```python
from build123d import *

# Parameters (mm, degrees)
SKETCH1_W                = 185
SKETCH1_H                = 70
SKETCH1_W_2              = 225
SKETCH1_H_2              = 30
BOSS_EXTRUDE1_DEPTH      = 380
CUT_EXTRUDE1_START       = -130
CUT_EXTRUDE1_OUTLINE_W   = 225
CUT_EXTRUDE1_OUTLINE_H   = 320
CUT_EXTRUDE1_OUTLINE_W_2 = 185
CUT_EXTRUDE1_DEPTH       = 130
SKETCH3_W                = 320
SKETCH3_H                = 30
CUT_EXTRUDE2_DEPTH       = 30
SKETCH4_W                = 320
SKETCH4_H                = 70
CUT_EXTRUDE3_DEPTH       = 245


# Read off the part's stored shape, not the designer's step: Cut-Extrude1
with BuildPart() as part:
    # Sketch1 → Boss-Extrude1 (new body)
    with BuildSketch(Plane.XY):
        Polygon((250, 25), (-5, 25), (-5, 65), (-250, 65), (-250, -65), (250, -65), align=None)
        with Locations((-127.5, 0)):
            Rectangle(SKETCH1_W, SKETCH1_H, mode=Mode.SUBTRACT)
        with Locations((107.5, -20)):
            Rectangle(SKETCH1_W_2, SKETCH1_H_2, mode=Mode.SUBTRACT)
    extrude(amount=BOSS_EXTRUDE1_DEPTH)

    # Cut-Extrude1 outline → Cut-Extrude1 (cut)
    with BuildSketch(Plane(origin=(0, 65, 0), x_dir=(1, 0, 0), z_dir=(0, 1, 0)).offset(CUT_EXTRUDE1_START)):
        with Locations((107.5, -190)):
            Rectangle(CUT_EXTRUDE1_OUTLINE_W, CUT_EXTRUDE1_OUTLINE_H)
        with Locations((-127.5, -190)):
            Rectangle(CUT_EXTRUDE1_OUTLINE_W_2, CUT_EXTRUDE1_OUTLINE_H)
    extrude(amount=CUT_EXTRUDE1_DEPTH, mode=Mode.SUBTRACT)

    # Sketch3 → Cut-Extrude2 (cut)
    with BuildSketch(Plane(origin=(250, 0, 0), x_dir=(0, 0, -1), z_dir=(1, 0, 0))):
        with Locations((-190, -20)):
            Rectangle(SKETCH3_W, SKETCH3_H)
    extrude(amount=-CUT_EXTRUDE2_DEPTH, mode=Mode.SUBTRACT)

    # Sketch4 → Cut-Extrude3 (cut)
    with BuildSketch(Plane.ZY.offset(250)):
        with Locations((190, 0)):
            Rectangle(SKETCH4_W, SKETCH4_H)
    extrude(amount=-CUT_EXTRUDE3_DEPTH, mode=Mode.SUBTRACT)


solid = part.part
```
Check sheet for the modelled part. Datum: model origin and axes. Units: mm. A direction names the side the tool comes from. Give positions to 0.01 mm unless a question says otherwise; leave off trailing zeros. Loops run counter-clockwise (first coordinate to the right, second up) from the corner with the lowest first, then second, coordinate; pieces in that order, holes last. Notation, with made-up numbers: (-21.75, -33) - (36.25, -33) arc R5 ccw to (36.25, -28) - close; hole circle Ø7 at (32, -3.75). An arc over 180 degrees is marked (long way). One line per question, with ' | ' between items. Start each with the question number.
1. Cross-section at B-B, the plane x = -116.5. Enter the section's corners in (y, z), plus the area to 3 significant figures.
2. Gauge pin test, flat ends, axial feed: pin 1 Ø24 at (x, z) = (87.5, 9) entering from +Y; pin 2 Ø12 at (x, y) = (23, -9.5) entering from +Z; pin 3 Ø4 at (y, z) = (7, 245) entering from -X. Record the tip position at first contact, or that the pin passes through.
3. Cross-section at A-A, the plane z = 313.5. Enter the section's corners in (x, y).
4. Set-up check for faces 1 (the flat face through (-20, -35, 188)), 2 (the flat face through (-129, -50, 30)), 3 (the flat face through (106, -5, 365)), 4 (the flat face through (-250, 44, 187)): record each of +Z, -Z, +X, -X, +Y, -Y from which the full face is reachable in a straight line by a thin tool's end or side.
5. Cross-section at C-C, the plane y = -29. Enter the section's corners in (x, z), plus the area to 3 significant figures.
6. Cross-section at D-D, the plane y = -56. Enter the section's corners in (x, z), plus the area to 3 significant figures.
7. Draft check along Y on faces 5 (the flat face through (-235, -35, 188)), 6 (the flat face through (220, -50, 192)), 7 (the flat face through (-35, 0, 15)), 8 (the flat face through (227, 25, 189)). Enter one of: released by +Y, released by -Y, zero draft, split by the parting line, or undercut.
8. Material ranges on line 1 along X through (y, z) = (-52.5, 209); line 2 along Z through (x, y) = (60, -45); line 3 along Y through (x, z) = (-14, 54), recorded low to high. Write a range as [from, to].
Check result:
1) outline: (-65, 0) - (-35, 0) - (-35, 30) - (-65, 30) - close; (-65, 350) - (-35, 350) - (-35, 380) - (-65, 380) - close; (35, 0) - (65, 0) - (65, 30) - (35, 30) - close; (35, 350) - (65, 350) - (65, 380) - (35, 380) - close | area: 3,600 mm2
2) pin 1: stops at y = 25 | pin 2: stops at z = 380 | pin 3: stops at x = 220
3) outline: (-250, -65) - (-220, -65) - (-220, -35) - (-250, -35) - close; (-250, 35) - (-220, 35) - (-220, 65) - (-250, 65) - close; (-35, -65) - (-5, -65) - (-5, -35) - (-35, -35) - close; (-35, 35) - (-5, 35) - (-5, 65) - (-35, 65) - close; (220, -65) - (250, -65) - (250, -35) - (220, -35) - close; (220, -5) - (250, -5) - (250, 25) - (220, 25) - close
4) face 1: +X, -X | face 2: +Y, -Y | face 3: +Z, -Z | face 4: +Z, -Z, -X, +Y, -Y
5) outline: (-250, 0) - (-220, 0) - (-220, 30) - (-250, 30) - close; (-250, 350) - (-220, 350) - (-220, 380) - (-250, 380) - close; (-35, 0) - (-5, 0) - (-5, 30) - (-35, 30) - close; (-35, 350) - (-5, 350) - (-5, 380) - (-35, 380) - close; (220, 0) - (250, 0) - (250, 30) - (220, 30) - close; (220, 350) - (250, 350) - (250, 380) - (220, 380) - close | area: 5,400 mm2
6) outline: (-250, 0) - (250, 0) - (250, 380) - (-250, 380) - close; hole (-220, 30) - (-35, 30) - (-35, 350) - (-220, 350) - close; hole (-5, 30) - (220, 30) - (220, 350) - (-5, 350) - close | area: 58,800 mm2
7) face 5: undercut | face 6: zero draft | face 7: undercut | face 8: released by +Y
8) line 1: x = [-250, -220], [-35, -5], [220, 250] | line 2: z = [0, 30], [350, 380] | line 3: y = [-65, -35], [35, 65]
